Verification items for the finished model (mm, model axes). Face numbers are marked on the shaded views. Give positions to 0.01 mm unless a question says otherwise; leave off trailing zeros. Write each loop counter-clockwise with the first axis right and the second up, starting at its lowest first coordinate (ties: lowest second). Pieces come first, ordered by that corner, then holes. Notation, with made-up numbers: M -25.75,-0.5 L 7.25,-0.5 A18 cw 7.25,15.5 Z; hole C -30,10.5 d5. An arc over 180 degrees is marked long. Write item = value, one per line.
Autodesk Inventor part; units mm, degrees
ref_plane "YZ Plane" through (0, 0, 0) normal (1, 0, 0) x (0, 1, 0)
ref_plane "XZ Plane" through (0, 0, 0) normal (0, 1, 0) x (-1, 0, 0)
ref_plane "XY Plane" through (0, 0, 0) normal (0, 0, 1) x (1, 0, 0)
sketch "Skizze1" plane through (0, 0, 0) normal (0, 0, 1) x (1, 0, 0)
  line L0 (-18.1618, 0.375) -> (-21.3761, 7.875)
  line L1 (-2.9476, 7.875) -> (-6.1618, 0.375)
  line L2 (-6.1618, 0.375) -> (-18.1618, 0.375)
  line L3 (-18.1618, 0.375) -> (-31.1618, 0.375)
  line L4 (-31.1618, 0.375) -> (-31.1618, 11.375)
  line L5 (-31.1618, 11.375) -> (6.8382, 11.375)
  line L6 (6.8382, 11.375) -> (6.8382, 0.375)
  line L7 (6.8382, 0.375) -> (-6.1618, 0.375)
  line L8 (-21.5376, 7.875) -> (-2.9476, 7.875)
  point P0 (0, 0)
  point P1 (-21.1618, 7.375)
  point P2 (-3.1618, 7.375)
  dimension "d10" = 38
  dimension "d14" = 12
  dimension "d29" = 13
extrude "Extrusion1" add sketch "Skizze1" along normal blind 50 contours L3 L4 L5 L6 L7 L1 L8 L0
sketch "Skizze2" plane through (6.8382, 0.375, 0) normal (1, 0, 0) x (0, 0, -1)
  line L0 (-50, 0) -> (-50, 11)
  line L1 (0, 11) -> (-50, 11)
  point P0 (0, -0.375)
  point P1 (-25, 4.85)
  dimension "d19" = 6.15
hole "Bohrung1" at (6.8382, 5.225, 25) direction (-1, 0, 0) diameter 2.9 depth 8 tip angle 118
sketch "Skizze3" plane through (-21.3761, 7.875, 0) normal (0, -1, 0) x (1, 0, 0)
  line L0 (0, 50) -> (18.4286, 50)
  line L1 (28.2143, 0) -> (28.2143, 50)
  point P0 (21.3761, 0)
sketch "Skizze4" plane through (-21.3761, 7.875, 0) normal (0, -1, 0) x (1, 0, 0)
  line L0 (0, 50) -> (18.4286, 50)
  line L1 (28.2143, 0) -> (28.2143, 50)
  point P0 (21.3761, 0)
  point P1 (9.2143, 25)
  dimension "d30" = 25
  dimension "d31" = 19
hole "Bohrung2" at (-12.1618, 7.875, 25) direction (0, 1, 0) diameter 5.2 end through all countersink diameter 10.5 countersink angle 90
properties part number "Schienenläuderaufsatz-22.11"
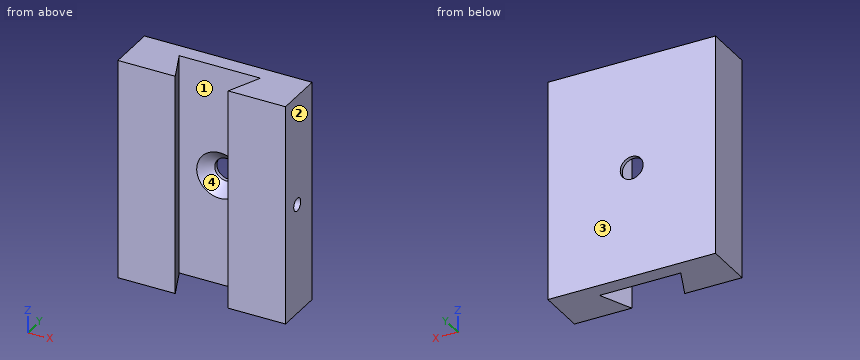
1) Depth check by flat-ended pin: P1, Ø4, axis at x = -12.16, z = 25, coming from the +Y side. Enter the tip coordinate at first touch or a pass-through.
From the geometry:
P1 = through
2) Cross-section at D-D on y = 9.5. Record the boundary of the cut face in (x, z) (3 decimals).
From the geometry:
outline = M -31.162,0 L 6.838,0 L 6.838,50 L -31.162,50 Z; hole C -12.162,25 d7.25
3) Cross-section at A-A on x = -19.5. Record the boundary of the cut face in (y, z) (3 decimals), plus the area to 3 significant figures.
From the geometry:
outline = M 0.375,0 L 3.497,0 L 3.497,50 L 0.375,50 Z; M 7.875,0 L 11.375,0 L 11.375,50 L 7.875,50 Z
area = 331 mm^2
4) Cross-section at B-B on y = 2. Record the boundary of the cut face in (x, z).
From the geometry:
outline = M -31.16,0 L -18.86,0 L -18.86,50 L -31.16,50 Z; M -5.47,0 L 6.84,0 L 6.84,50 L -5.47,50 Z
5) Cross-section at C-C on z = 43.5. Record the boundary of the cut face in (x, y) (3 decimals), plus the area to 3 significant figures.
From the geometry:
outline = M -31.162,0.375 L -18.162,0.375 L -21.376,7.875 L -2.948,7.875 L -6.162,0.375 L 6.838,0.375 L 6.838,11.375 L -31.162,11.375 Z
area = 304 mm^2
6) Draft check along X on the marked faces 1, 2, 3 and 4. Enter one of: +X half, -X half, draft (parallel to the pull), parting line (faces both ways), or undercut.
From the geometry:
face_1 = undercut
face_2 = +X half
face_3 = draft
face_4 = undercut
7) Material ranges on probe 1 along Y at (x, z) = (0.75, 25) (3 decimals); probe 2 along X at (y, z) = (10.8, 25); probe 3 along Y at (x, z) = (-18, 4) (3 decimals), recorded low to high. Write a range as from..to.
From the geometry:
probe_1 = 0.375..3.775, 6.675..11.375
probe_2 = -31.16..-14.76, -9.56..6.84
probe_3 = 7.875..11.375
